Can you work these out from the model? Positions are in its coordinate system, mm. A direction names the side the tool comes from. Coordinates: 2 decimals unless noted, no trailing zeros. Loops run counter-clockwise (first coordinate to the right, second up) from the corner with the lowest first, then second, coordinate; pieces in that order, holes last. Notation, with made-up numbers: (56, -36.5) -> (101, -36.5) arc R23 cw to (101, -23.5) -> close; hole circle Ø10 at (41.25, 62). An arc over 180 degrees is marked (long way). Use one line per item in the form item = value. Start each with the question number.
(1) Imagine slicing it at A-A (y = 6). List the corners of the cut face in (x, z) for me, plus the area to 3 significant figures.
(2) Thinking about a two-plate mould opening in X: for faces 1 (the flat face through (-40, 1, -3.95)), 2 (the cylindrical face through (-67.1, 1.23, -88.09)), 3 (the cylindrical face through (-63.013, 4.719, -85.645)), which applies, released by +X, released by -X, zero draft, split by the parting line, or undercut?
(3) On a 3-axis mill with a long thin cutter (end or side, diameter ignored), from which of +Z, -Z, +X, -X, +Y, -Y can I reach the whole of each face in a straight line? I mean faces 4 (the flat face through (-66, 7.5, -29)), 5 (the cylindrical face through (-63.013, 4.719, -27.645)). Say none if no direction works.
(4) Imagine slicing it at C-C (x = -41). List the corners of the cut face in (y, z) for me, plus the area to 4 significant figures.
(5) Imagine slicing it at B-B (z = -67.5). List the corners of the cut face in (x, y) for me.
(6) I'm going to push flat-ended pins straight in: pin 1 (3 mm diameter, centred on x = -27.5, z = -53, fed in from -Y); pin 2 (1.5 mm diameter, centred on x = -64.5, z = -28, fed in from +Y). Where does each tip first touch, or does it pass through?
(7) I need wall thicknesses on line 1 (Z direction, x = -64.5, y = 3.6); line 2 (X direction, y = 4.1, z = -85.45); line 3 (Y direction, x = -35.5, z = -26.5). Which ranges of each line are inside material? Lowest first, please. Write a range as [from, to].
```python
from build123d import *

# Parameters (mm, degrees)
BOSS_EXTRUDE1_DEPTH = 2.5
SKETCH3_R           = 3.5
SKETCH3_R_2         = 1.5
BOSS_EXTRUDE2_DEPTH = 5
CHAMFER1_SIZE       = 0.5


with BuildPart() as part:
    # Sketch2 → Boss-Extrude1 (new body)
    with BuildSketch(Plane(origin=(0, 0, 0), x_dir=(1, 0, 0), z_dir=(0, 1, 0))):
        with BuildLine():
            Line((-68, 85.95), (-68, 6.95))
            ThreePointArc((-68, 6.95), (-67.121320344, 4.828679656), (-65, 3.95))
            Line((-65, 3.95), (-15, 3.95))
            ThreePointArc((-15, 3.95), (-12.878679656, 4.828679656), (-12, 6.95))
            Line((-12, 6.95), (-12, 85.95))
            ThreePointArc((-12, 85.95), (-12.878679656, 88.071320344), (-15, 88.95))
            Line((-15, 88.95), (-65, 88.95))
            ThreePointArc((-65, 88.95), (-67.121320344, 88.071320344), (-68, 85.95))
        make_face()
    extrude(amount=BOSS_EXTRUDE1_DEPTH)

    # Sketch3 → Boss-Extrude2 (add)
    # profile 1 of 4: a face of its own
    with BuildSketch(Plane(origin=(0, 2.5, 0), x_dir=(1, 0, 0), z_dir=(0, 1, 0))):
        with Locations(Location((-64.5, 85.45, 0), (0, 0, 90))):
            Circle(SKETCH3_R)
        with Locations(Location((-64.5, 85.45, 0), (0, 0, 270))):
            Circle(SKETCH3_R_2, mode=Mode.SUBTRACT)
    # profile 2 of 4: a face of its own
    with BuildSketch(Plane(origin=(0, 2.5, 0), x_dir=(1, 0, 0), z_dir=(0, 1, 0))):
        with Locations(Location((-15.5, 85.45, 0), (0, 0, 90))):
            Circle(SKETCH3_R)
        with Locations(Location((-15.5, 85.45, 0), (0, 0, 270))):
            Circle(SKETCH3_R_2, mode=Mode.SUBTRACT)
    # profile 3 of 4: a face of its own
    with BuildSketch(Plane(origin=(0, 2.5, 0), x_dir=(1, 0, 0), z_dir=(0, 1, 0))):
        with Locations((-15.5, 27.45)):
            Circle(SKETCH3_R)
        with Locations(Location((-15.5, 27.45, 0), (0, 0, 270))):
            Circle(SKETCH3_R_2, mode=Mode.SUBTRACT)
    # profile 4 of 4: a face of its own
    with BuildSketch(Plane(origin=(0, 2.5, 0), x_dir=(1, 0, 0), z_dir=(0, 1, 0))):
        with Locations(Location((-64.5, 27.45, 0), (0, 0, 180))):
            Circle(SKETCH3_R)
        with Locations(Location((-64.5, 27.45, 0), (0, 0, 270))):
            Circle(SKETCH3_R_2, mode=Mode.SUBTRACT)
    extrude(amount=BOSS_EXTRUDE2_DEPTH)

    # Chamfer1
    chamfer1_edges = [part.edges().sort_by_distance(p)[0] for p in [
        (-64.5, 7.5, -86.95),
        (-15.5, 7.5, -86.95),
        (-15.5, 7.5, -28.95),
        (-64.5, 7.5, -28.95),
    ]]
    chamfer(chamfer1_edges, length=CHAMFER1_SIZE)


solid = part.part
```
Worked out:
q1.outline = circle Ø7 at (-64.5, -85.45); circle Ø7 at (-64.5, -27.45); circle Ø7 at (-15.5, -85.45); circle Ø7 at (-15.5, -27.45); hole circle Ø3 at (-64.5, -85.45); hole circle Ø3 at (-64.5, -27.45); hole circle Ø3 at (-15.5, -85.45); hole circle Ø3 at (-15.5, -27.45)
q1.area = 126 mm2
q2.face_1 = zero draft
q2.face_2 = released by -X
q2.face_3 = undercut
q3.face_4 = +Z, -Z, +X, -X, +Y
q3.face_5 = +Y
q4.outline = (0, -88.95) -> (2.5, -88.95) -> (2.5, -3.95) -> (0, -3.95) -> close
q4.area = 212.5 mm2
q5.outline = (-68, 0) -> (-12, 0) -> (-12, 2.5) -> (-68, 2.5) -> close
q6.pin_1 = 0
q6.pin_2 = 2.5
q7.line_1 = [-88.95, -86.95], [-83.95, -81.95], [-30.95, -28.95], [-25.95, -23.95]
q7.line_2 = [-68, -66], [-63, -61], [-19, -17], [-14, -12]
q7.line_3 = [0, 2.5]
